Work out the finished part from the listing and answer in its coordinate system (mm). A direction names the side the tool comes from. Coordinates: 2 decimals unless noted, no trailing zeros. Loops run counter-clockwise (first coordinate to the right, second up) from the corner with the lowest first, then second, coordinate; pieces in that order, holes last. Notation, with made-up numbers: M 52,-17 L 80,-17 A21 ccw 80,-6 Z; hole C 75,22 d5. An arc over 180 degrees is marked long. Write each question's results on one line, items separated by ' | '.
```python
from build123d import *

# Parameters (mm, degrees)
SKETCH1_W           = 154
SKETCH1_H           = 26
SKETCH1_R           = 1.7
BOSS_EXTRUDE1_DEPTH = 4
SKETCH3_W           = 10.3
SKETCH3_H           = 15
BOSS_EXTRUDE2_DEPTH = 24
CHAMFER2_SIZE       = 7
CHAMFER2_SIZE2      = 19.232341936
CHAMFER3_SIZE       = 7
CHAMFER3_SIZE_2     = 19.232341936
SKETCH4_W           = 10
SKETCH4_H           = 10
CUT_EXTRUDE1_DEPTH  = 24
SKETCH6_R           = 1.7
CUT_EXTRUDE2_DEPTH  = 15


with BuildPart() as part:
    # Sketch1 → Boss-Extrude1 (new body)
    with BuildSketch(Plane(origin=(0, 0, 0), x_dir=(1, 0, 0), z_dir=(0, 1, 0))):
        with Locations((0, 66)):
            Rectangle(SKETCH1_W, SKETCH1_H)
        with Locations(Location((72, 66, 0), (0, 0, 270))):
            Circle(SKETCH1_R, mode=Mode.SUBTRACT)
        with Locations(Location((-72, 66, 0), (0, 0, 270))):
            Circle(SKETCH1_R, mode=Mode.SUBTRACT)
    extrude(amount=BOSS_EXTRUDE1_DEPTH)

    # Sketch3 → Boss-Extrude2 (add)
    with BuildSketch(Plane(origin=(0, 4, 0), x_dir=(1, 0, 0), z_dir=(0, 1, 0))):
        with Locations((-61.85, 66.2)):
            Rectangle(SKETCH3_W, SKETCH3_H)
        with Locations((-10.85, 66.2)):
            Rectangle(SKETCH3_W, SKETCH3_H)
    extrude(amount=BOSS_EXTRUDE2_DEPTH)

    # Chamfer2
    chamfer2_edges = [part.edges().sort_by_distance(p)[0] for p in [
        (-5.7, 4, -66.2),
    ]]
    chamfer2_side = [part.faces().sort_by_distance(p)[0] for p in [
        (3.054836525, 4, -65.983192096),
    ]]
    chamfer(chamfer2_edges, length=CHAMFER2_SIZE, length2=CHAMFER2_SIZE2, reference=chamfer2_side[0])

    # Chamfer3
    # the kernel refuses this chamfer: 19.232341936, 7 mm, written as the material it adds along each edge
    with BuildSketch(Plane(origin=(-67, 4, -73.7), x_dir=(-0.9950833631817486, -0.09904090225205066, 0), z_dir=(0, 0, 1))) as chamfer3_piece_1_section:
        Polygon((CHAMFER3_SIZE * 0.995083363182, -CHAMFER3_SIZE * 0.0990409022521), (-CHAMFER3_SIZE_2 * 0.099040902253, -CHAMFER3_SIZE_2 * 0.995083363191), (0, 0), align=None)
    chamfer3_piece_1 = extrude(amount=15, mode=Mode.PRIVATE)
    chamfer3_piece_1 = chamfer3_piece_1 - Plane(origin=(-72, 10.759738183, -66), x_dir=(0, 0, 1), z_dir=(0, -1, 0)) * Cylinder(1.7, 107, mode=Mode.PRIVATE)
    add(chamfer3_piece_1)

    # Sketch4 → Cut-Extrude1 (cut)
    with BuildSketch(Plane(origin=(0, 28, 0), x_dir=(1, 0, 0), z_dir=(0, 1, 0))):
        with Locations((-72, 66)):
            Rectangle(SKETCH4_W, SKETCH4_H)
    extrude(amount=-CUT_EXTRUDE1_DEPTH, mode=Mode.SUBTRACT)

    # Sketch6 → Cut-Extrude2 (cut)
    with BuildSketch(Plane.XY.offset(-58.7)):
        with Locations((-60.35, 9.1)):
            Circle(SKETCH6_R)
        with Locations((-60.35, 19.1)):
            Circle(SKETCH6_R)
        with Locations((-12.35, 9.1)):
            Circle(SKETCH6_R)
        with Locations((-12.35, 19.1)):
            Circle(SKETCH6_R)
    extrude(amount=-CUT_EXTRUDE2_DEPTH, mode=Mode.SUBTRACT)


solid = part.part
```
1) Straight lines are drawn through the part: probe 1 along X at (y, z) = (0.95, -66); probe 2 along Y at (x, z) = (-12.35, -63.25); probe 3 along X at (y, z) = (19.5, -69.75). For each, find the intervals that lie inside material, in ascending order. Write a range as [from, to].
Check result:
probe 1: [-77, -73.7], [-70.3, 70.3], [73.7, 77] | probe 2: [0, 7.4], [10.8, 17.4], [20.8, 28] | probe 3: [-67, -62], [-58.7, -56.7], [-16, -14], [-10.7, -4.34]
2) Find section C-C, the plane y = 25.5. Give the vertices of the cut face in (x, z), and give its area (3 significant figures).
Check result:
outline: M -67,-73.7 L -56.7,-73.7 L -56.7,-58.7 L -67,-58.7 Z; M -16,-73.7 L -5.7,-73.7 L -5.7,-58.7 L -16,-58.7 Z | area: 309 mm^2
3) Given pin 1 Ø1.5 at (y, z) = (8.5, -69.5) entering from -X; pin 2 Ø7.5 at (x, y) = (-71.5, 18) entering from +Z; pin 3 Ø5 at (x, y) = (-67.5, 18) entering from -Z, each flat-ended and moving along its own axis, determine where each tip first touches the part or whether it passes through.
Check result:
pin 1: x = -67 | pin 2: z = -58.7 | pin 3: z = -73.7
4) Find section B-B, the plane x = -12.35. Give the vertices of the cut face in (y, z).
Check result:
outline: M 0,-79 L 4,-79 L 4,-73.7 L 7.4,-73.7 L 7.4,-58.7 L 4,-58.7 L 4,-53 L 0,-53 Z; M 10.8,-73.7 L 17.4,-73.7 L 17.4,-58.7 L 10.8,-58.7 Z; M 20.8,-73.7 L 28,-73.7 L 28,-58.7 L 20.8,-58.7 Z
5) Find section D-D, the plane x = 72. Give the vertices of the cut face in (y, z).
Check result:
outline: M 0,-79 L 4,-79 L 4,-67.7 L 0,-67.7 Z; M 0,-64.3 L 4,-64.3 L 4,-53 L 0,-53 Z
6) For a pull along Y with two mould halves and no side action, classify faces 5 (the face through (-59.57, 17.59, -66.1)), 6 (the face through (-5.7, 26, -66)), 7 (the face through (-2.25, 13.75, -66.1)) as released by +Y, released by -Y, zero draft, split by the parting line, or undercut.
Check result:
face 5: undercut | face 6: zero draft | face 7: released by +Y
7) Find section A-A, the plane z = -66. Give the vertices of the cut face in (x, y).
Check result:
outline: M -77,0 L -73.7,0 L -73.7,4 L -77,4 Z; M -70.3,0 L 70.3,0 L 70.3,4 L 1.3,4 L -5.7,23.23 L -5.7,28 L -16,28 L -16,4 L -56.7,4 L -56.7,28 L -67,28 L -67,4 L -70.3,4 Z; M 73.7,0 L 77,0 L 77,4 L 73.7,4 Z; hole C -60.35,9.1 d3.4; hole C -60.35,19.1 d3.4; hole C -12.35,9.1 d3.4; hole C -12.35,19.1 d3.4
8) Which of the six approach directions +Z, -Z, +X, -X, +Y, -Y give full straight-line access (tool end or side, diameter ignored) to faces 1 (the face through (-69, 9, -61)), 2 (the face through (-63, 16, -73.7)), 3 (the face through (-16, 16, -66)), 4 (the face through (-9, 16, -58.7))?
Check result:
face 1: -X, +Y | face 2: -Z, +X, -X, +Y | face 3: +Z, -Z, +Y | face 4: +Z, +X, -X, +Y
